Autodesk Inventor part; units mm, degrees
ref_plane "YZ Plane" through (0, 0, 0) normal (1, 0, 0) x (0, 1, 0)
ref_plane "XZ Plane" through (0, 0, 0) normal (0, 1, 0) x (-1, 0, 0)
ref_plane "XY Plane" through (0, 0, 0) normal (0, 0, 1) x (1, 0, 0)
sketch "Skizze1" plane through (0, 0, 0) normal (0, 0, 1) x (1, 0, 0)
  line L0 (-15, 5) -> (15, 5)
  line L1 (15, 5) -> (15, 0)
  line L2 (-15, 0) -> (-15, 5)
  line L3 (26.2, 0) -> (26.2, -10)
  line L4 (26.2, -10) -> (-26.2, -10)
  line L5 (-26.2, -10) -> (-26.2, 0)
  line L6 (-26.2, 0) -> (-15, 0)
  line L7 (15, 0) -> (26.2, 0)
  line L8 (0, 8) -> (0, -13)
  point P0 (0, 0)
  dimension "d0" = 30
  dimension "d1" = 5
  dimension "d2" = 52.4
  dimension "d3" = 10
extrude "Extrusion1" add sketch "Skizze1" along normal blind 1
sketch "Skizze3" plane through (0, 0, 1) normal (0, 0, 1) x (1, 0, 0)
  line L0 (0, 8) -> (0, -13)
  line L1 (-36.68, 0) -> (36.68, 0)
  point P0 (0, 0)
  point P1 (22.05, -8)
  point P2 (-22.05, -8)
  dimension "d18" = 22.05
  dimension "d19" = 8
hole "Bohrung2" at (22.05, -8, 1) at (-22.05, -8, 1) direction (0, 0, -1) diameter 2.1 end through all
sketch "Skizze4" plane through (0, 0, 0) normal (0, 0, -1) x (-1, 0, 0)
  line L0 (-2.05, 4.6) -> (-3.45, 4.6)
  line L1 (-3.45, 4.6) -> (-3.45, 1.6)
  line L2 (-3.45, 1.6) -> (-2.05, 1.6)
  line L3 (-2.05, 1.6) -> (-2.05, 4.6)
  line L4 (15, 5) -> (-15, 5)
  line L5 (0, -13) -> (0, 8)
  line L6 (-2.75, 4.6) -> (-2.75, 1.6) construction
  point P0 (0, 0)
  dimension "d27" = 1.4
  dimension "d28" = 0.4
  dimension "d29" = 3
  dimension "d31" = 2.75
extrude "Extrusion2" add sketch "Skizze4" along normal blind 0.05
pattern_linear "Rechteckige Anordnung2" count 6 spacing 2 along (1, 0, 0) of "Extrusion2"
mirror "Spiegeln2" about plane through (0, 0, 0) normal (1, 0, 0) of "Extrusion2", "Rechteckige Anordnung2"
properties part number "Ballsensor IR Platine" material "Phenolharz"
Source: CAD feature listing. Evaluate the final solid. Frame: model axes, mm. A direction names the side the tool comes from. Round coordinates to 2 decimals unless told otherwise and drop trailing zeros. Loops run counter-clockwise (first coordinate to the right, second up) from the corner with the lowest first, then second, coordinate; pieces in that order, holes last.
(1) Section query C-C (z = 0.35). Output: boundary loops of the cut face in (x, y).
From the geometry:
outline: (-26.2, -10) - (26.2, -10) - (26.2, 0) - (15, 0) - (15, 5) - (-15, 5) - (-15, 0) - (-26.2, 0) - close; hole circle Ø2.1 at (-22.05, -8); hole circle Ø2.1 at (22.05, -8)
(2) Section query A-A (y = -8). Output: boundary loops of the cut face in (x, z), and give its area (3 significant figures).
From the geometry:
outline: (-26.2, 0) - (-23.1, 0) - (-23.1, 1) - (-26.2, 1) - close; (-21, 0) - (21, 0) - (21, 1) - (-21, 1) - close; (23.1, 0) - (26.2, 0) - (26.2, 1) - (23.1, 1) - close
area: 48.2 mm2
(3) Pull-direction query (X, two-part tool) for faces 4 (the flat face through (9, 3, -0.05)), 5 (the cylindrical face through (-21.025, -7.772, 0.493)), 6 (the cylindrical face through (21.01, -7.86, 0.49)), 7 (the flat face through (-15, 2.5, 0.5)); classes: +X half, -X half, draft (parallel to the pull), parting line (faces both ways), or undercut.
From the geometry:
face 4: draft
face 5: undercut
face 6: undercut
face 7: -X half
(4) Section query B-B (x = -22.05). Output: boundary loops of the cut face in (y, z).
From the geometry:
outline: (-10, 0) - (-9.05, 0) - (-9.05, 1) - (-10, 1) - close; (-6.95, 0) - (0, 0) - (0, 1) - (-6.95, 1) - close
(5) Section query D-D (x = -7). Output: boundary loops of the cut face in (y, z), and give its area (4 significant figures).
From the geometry:
outline: (-10, 0) - (1.6, 0) - (1.6, -0.05) - (4.6, -0.05) - (4.6, 0) - (5, 0) - (5, 1) - (-10, 1) - close
area: 15.15 mm2
(6) Access query for faces 1 (the flat face through (-20.7, 0, 0.5)), 2 (the flat face through (26.2, -4.9, 0.5)), 3 (the flat face through (15, 2.5, 0.5)). Directions: +Z, -Z, +X, -X, +Y, -Y. A direction counts if a zero-diameter tool reaches every point of the face in a straight line with its end or side. Return the directions, or none.
From the geometry:
face 1: +Z, -Z, -X, +Y
face 2: +Z, -Z, +X, +Y, -Y
face 3: +Z, -Z, +X, +Y
(7) Contact query for a flat-ended pin moving along its axis: pin 1 Ø6 at (x, y) = (-15, -2.5) entering from -Z. Output: stop coordinate, or through.
From the geometry:
pin 1: stops at z = 0
(8) Material intervals for probe 1 along X at (y, z) = (-8, 0.25); probe 2 along Y at (x, z) = (22.05, 0.55); probe 3 along Z at (x, y) = (-9, 1.5), sorted ascending.
From the geometry:
probe 1: x = -26.2 to -23.1, -21 to 21, 23.1 to 26.2
probe 2: y = -10 to -9.05, -6.95 to 0
probe 3: z = 0 to 1
